Source: CAD feature listing. Evaluate the final solid. Frame: model axes, mm. A direction names the side the tool comes from. Coordinates: 2 decimals unless noted, no trailing zeros. Order: outer loops, then holes, each group sorted by start corner. A loop starts at its lowest first (then second) coordinate and runs counter-clockwise, first axis right, second up.
Item 1: Section A-A on z = -8.5. Return the cut outline in (x, y), then the cut area to 3 significant figures.
Item 2: Contact query for flat-ended pins moving along their axis: P1, Ø1.5, axis at x = 0, y = -3.5, coming from the +Z side; P2, Ø0.6, axis at x = 5.5, y = -9.5, coming from the -Z side; P3, Ø0.8, axis at x = -4.5, z = -8.5, coming from the -Y side; P4, Ø1.5, axis at x = 5.5, z = -6, coming from the +Y side. Output: stop coordinate, or through.
Item 3: Ray query, line 1 (X direction, y = -7.25, z = -7); line 2 (X direction, y = -9.25, z = -5.25); line 3 (Z direction, x = 0, y = -2.5). Return the intervals inside material, ascending.
Item 4: Mould query, pull axis X, two halves, no side actions, for faces 1 (the flat face through (-6.85, -7, -5)), 2 (the flat face through (-3.25, -7, -7)), 3 (the flat face through (0, -5, 0)), 4 (the cylindrical face through (5.7, -2.02, -5.44)). Classes: released by +X, released by -X, zero draft, split by the parting line, or undercut.
Item 5: Section D-D on z = -2.75. Return the cut outline in (x, y).
Item 6: Reachability of faces 5 (the flat face through (5, -8.8, -8)), 6 (the cylindrical face through (-5.628, -1.995, -5.437)), 7 (the flat face through (5, -5, -9)) from +Z, -Z, +X, -X, +Y, -Y: full face, straight path, thin tool, end or side. Return the list, or none.
Item 7: Section B-B on z = -6.75. Return the cut outline in (x, y).
Item 8: Section C-C on x = 5.5. Return the cut outline in (y, z), then the cut area to 3 significant figures.
from build123d import *

# Parameters (mm, degrees)
PAD_DEPTH       = 10
POCKET_DEPTH    = 9
POCKET001_DEPTH = 1.2
SKETCH009_W     = 13.7
SKETCH009_H     = 10
PAD001_DEPTH    = 10


with BuildPart() as obj1:
    # Sketch → Pad (new body)
    with BuildSketch(Plane.XZ):
        with BuildLine():
            ThreePointArc((-6.827152, 0), (0, -5.9), (6.827152, 0))
            Line((8, 0), (6.827152, 0))
            Line((8, -10), (8, 0))
            Line((-8, -10), (8, -10))
            Line((-8, 0), (-8, -10))
            Line((-6.827152, 0), (-8, 0))
        make_face()
    extrude(amount=PAD_DEPTH)

    # Sketch007 → Pocket (cut)
    with BuildSketch(Plane.XY):
        with BuildLine():
            Line((-6.85, -3.7), (-6.85, -8.8))
            Line((-6.85, -8.8), (-3.25, -8.8))
            Line((-3.25, -8.8), (-3.25, -3.7))
            ThreePointArc((-3.25, -3.7), (-5.05, -1.9), (-6.85, -3.7))
        make_face()
        with BuildLine():
            Line((3.25, -3.7), (3.25, -8.8))
            Line((3.25, -8.8), (6.85, -8.8))
            Line((6.85, -8.8), (6.85, -3.7))
            ThreePointArc((6.85, -3.7), (5.05, -1.9), (3.25, -3.7))
        make_face()
    extrude(amount=-POCKET_DEPTH, mode=Mode.SUBTRACT)

    # Sketch008 (on Face7 of Pocket) → Pocket001 (cut)
    with BuildSketch(Plane.XZ.offset(10)):
        Polygon((-6.85, 0), (-6.85, -7.3), (-3.25, -7.3), (-3.25, -2), (3.25, -2), (3.25, -7.3), (6.85, -7.3), (6.85, 0), align=None)
    extrude(amount=-POCKET001_DEPTH, mode=Mode.SUBTRACT)


with BuildPart() as body001:
    # Sketch009 (on ShapeBinder) → Pad001 (new body)
    with BuildSketch(Plane.XZ.offset(10)):
        with Locations((0, -5)):
            Rectangle(SKETCH009_W, SKETCH009_H)
    extrude(amount=-PAD001_DEPTH)

    # Boolean: cut obj1
    add(obj1.part, mode=Mode.SUBTRACT)


solid = body001.part
Answer list:
1. outline: (-6.85, -8.8) - (-3.25, -8.8) - (-3.25, -3.7) arc R1.8 ccw to (-6.85, -3.7) - close; (3.25, -8.8) - (6.85, -8.8) - (6.85, -3.7) arc R1.8 ccw to (3.25, -3.7) - close
1. area: 46.9 mm2
2. P1: stops at z = 0
2. P2: stops at z = -7.3
2. P3: stops at y = -8.8
2. P4: stops at y = -1.9
3. line 1: x = -6.85 to -3.25, 3.25 to 6.85
3. line 2: x = -6.85 to -3.25, -2.92 to 2.92, 3.25 to 6.85
3. line 3: z = -5.9 to 0
4. face 1: released by -X
4. face 2: undercut
4. face 3: zero draft
4. face 4: undercut
5. outline: (-6.85, -10) - (6.85, -10) - (6.85, -3.7) arc R1.8 ccw to (5.79, -2.06) - (5.79, 0) - (-5.79, 0) - (-5.79, -2.06) arc R1.8 ccw to (-6.85, -3.7) - close
6. face 5: -Z, +X, -X, -Y
6. face 6: -Z, +Y
6. face 7: -Z, +X, -X, +Y, -Y
7. outline: (-6.85, -10) - (-3.25, -10) - (-3.25, -3.7) arc R1.8 ccw to (-6.85, -3.7) - close; (3.25, -10) - (6.85, -10) - (6.85, -3.7) arc R1.8 ccw to (3.25, -3.7) - close
8. outline: (-10, -7.3) - (-8.8, -7.3) - (-8.8, -9) - (-1.96, -9) - (-1.96, -3.17) - (0, -3.17) - (0, 0) - (-10, 0) - close
8. area: 76.5 mm2
